Part model, mm, in its own coordinate system. A direction names the side the tool comes from. Coordinates: 2 decimals unless noted, no trailing zeros. Write each loop counter-clockwise with the first axis right and the second up, starting at its lowest first coordinate (ties: lowest second). Pieces come first, ordered by that corner, then holes. Notation, with made-up numbers: (19, -35.5) -> (67, -35.5) arc R20 ccw to (67, -15.5) -> close; hole circle Ø1 at (30.5, -8). An arc over 180 degrees is marked (long way). One line per question, with ' | ' between items. Start each with the question number.
Item 1: 3-axis set-ups, long thin cutter, end or side, ignore diameter. For faces 1 (the flat face through (0, 4, 18)), 2 (the cylindrical face through (-1.67, 6.17, 5.3)), 3 (the flat face through (3, 1.588, -3)): which of +Z, -Z, +X, -X, +Y, -Y reach the whole face in a straight line?
Item 2: Saw through at D-D (x = -14.5). List the corners of the cut face in (y, z).
Item 3: Saw through at A-A (x = 0). List the corners of the cut face in (y, z).
Item 4: Saw through at C-C (z = 0). List the corners of the cut face in (x, y).
Item 5: Probe probe 1 along Z at (x, y) = (12.7, 2); probe 2 along Z at (x, y) = (0, 2.25). List the from-to ranges inside material, lowest first. Write a range as [from, to].
Item 6: Two-plate mould, pull along X, no slides. Class faces 4 (the flat face through (-18, 4, 0)), 5 (the cylindrical face through (-13.375, 3.913, -10.556)), 6 (the flat face through (0, 7.938, 8)): pulls with the +X half, pulls with the -X half, needs draft (parallel to the pull), parting line crosses it, or undercut.
Item 7: Pin check, flat tips, straight feed: pin 1 (10 mm diameter, centred on x = 0, z = 0, fed in from +Y); pin 2 (2.5 mm diameter, centred on x = 12.7, z = 12.7, fed in from +Y). Stop position of each tip, or through.
Item 8: Saw through at B-B (y = 5.5). List the corners of the cut face in (x, z).
Autodesk Inventor part; units mm, degrees
ref_plane "YZ Plane" through (0, 0, 0) normal (1, 0, 0) x (0, 1, 0)
ref_plane "XZ Plane" through (0, 0, 0) normal (0, 1, 0) x (-1, 0, 0)
ref_plane "XY Plane" through (0, 0, 0) normal (0, 0, 1) x (1, 0, 0)
sketch "Sketch1" plane through (0, 0, 0) normal (0, 1, 0) x (-1, 0, 0)
  line L0 (-18, 18) -> (18, 18)
  line L1 (18, 18) -> (18, -18)
  line L2 (18, -18) -> (-18, -18)
  line L3 (-18, -18) -> (-18, 18)
  line L4 (-18, 18) -> (18, -18) construction
  line L5 (18, 18) -> (-18, -18) construction
  point P0 (0, 0)
  dimension "d0" = 36
  dimension "d1" = 36
extrude "Extrusion1" add sketch "Sketch1" along normal blind 7.9375
sketch "Sketch3" plane through (0, 7.9375, 0) normal (0, 1, 0) x (1, 0, 0)
  line L0 (-12.7, -12.7) -> (12.7, -12.7) construction
  line L1 (12.7, -12.7) -> (12.7, 12.7) construction
  line L2 (12.7, 12.7) -> (-12.7, 12.7) construction
  line L3 (-12.7, 12.7) -> (-12.7, -12.7) construction
  line L4 (-12.7, -12.7) -> (12.7, 12.7) construction
  line L5 (12.7, -12.7) -> (-12.7, 12.7) construction
  point P0 (0, 0)
  dimension "d11" = 25.4
hole "Hole2" at (-12.7, 7.9375, -12.7) at (12.7, 7.9375, -12.7) at (-12.7, 7.9375, 12.7) at (12.7, 7.9375, 12.7) direction (0, -1, 0) diameter 4.496 depth 12.3 tip angle 118
sketch "Sketch2" plane through (0, 7.9375, 0) normal (0, 1, 0) x (1, 0, 0)
  point P0 (0, 0)
  point P1 (0, 0)
hole "Hole1" at (0, 7.9375, 0) direction (0, -1, 0) diameter 6.528 end through all counterbore diameter 11.113 counterbore depth 3.25
fillet "Fillet1" radius 0.25 12 edges at (-18, 3.9688, 18) (0, 0, 18) (18, 3.9688, 18) (0, 7.9375, 18) (18, 7.9375, 0) (0, 7.9375, -18) (-18, 7.9375, 0) (18, 0, 0) (18, 3.9688, -18) (-18, 0, 0) (0, 0, -18) (-18, 3.9688, -18)
fillet "Fillet2" radius 0.25 1 edges at (0, 7.9375, -5.5565)
sketch "Sketch4" plane through (0, 0, 0) normal (0, -1, 0) x (1, 0, 0)
  circle A0 centre (0, 0) radius 12.687
  dimension "d21" = 25.374
extrude "Extrusion2" cut sketch "Sketch4" against normal blind 1.5875
properties part number "ball-holder-to-post-adapter" material "ABS Plastic"
From the geometry:
1) face 1: +Z, +X, -X, +Y, -Y | face 2: +Y | face 3: -Y
2) outline: (0, -17.75) arc R0.25 ccw to (0.25, -18) -> (7.69, -18) arc R0.25 ccw to (7.94, -17.75) -> (7.94, -14.05) -> (0, -14.05) -> close; (0, -11.35) -> (7.94, -11.35) -> (7.94, 11.35) -> (0, 11.35) -> close; (0, 14.05) -> (7.94, 14.05) -> (7.94, 17.75) arc R0.25 ccw to (7.69, 18) -> (0.25, 18) arc R0.25 ccw to (0, 17.75) -> close
3) outline: (0, -17.75) arc R0.25 ccw to (0.25, -18) -> (7.69, -18) arc R0.25 ccw to (7.94, -17.75) -> (7.94, -5.81) arc R0.25 ccw to (7.69, -5.56) -> (4.69, -5.56) -> (4.69, -3.26) -> (1.59, -3.26) -> (1.59, -12.69) -> (0, -12.69) -> close; (0, 12.69) -> (1.59, 12.69) -> (1.59, 3.26) -> (4.69, 3.26) -> (4.69, 5.56) -> (7.69, 5.56) arc R0.25 ccw to (7.94, 5.81) -> (7.94, 17.75) arc R0.25 ccw to (7.69, 18) -> (0.25, 18) arc R0.25 ccw to (0, 17.75) -> close
4) outline: (-18, 0.25) arc R0.25 ccw to (-17.75, 0) -> (-12.69, 0) -> (-12.69, 1.59) -> (-3.26, 1.59) -> (-3.26, 4.69) -> (-5.56, 4.69) -> (-5.56, 7.69) arc R0.25 ccw to (-5.81, 7.94) -> (-17.75, 7.94) arc R0.25 ccw to (-18, 7.69) -> close; (3.26, 1.59) -> (12.69, 1.59) -> (12.69, 0) -> (17.75, 0) arc R0.25 ccw to (18, 0.25) -> (18, 7.69) arc R0.25 ccw to (17.75, 7.94) -> (5.81, 7.94) arc R0.25 ccw to (5.56, 7.69) -> (5.56, 4.69) -> (3.26, 4.69) -> close
5) probe 1: [-18, -14.95], [-10.45, 10.45], [14.95, 18] | probe 2: [-18, -3.26], [3.26, 18]
6) face 4: pulls with the -X half | face 5: undercut | face 6: needs draft
7) pin 1: y = 4.69 | pin 2: through
8) outline: (-18, -17.75) arc R0.25 ccw to (-17.75, -18) -> (17.75, -18) arc R0.25 ccw to (18, -17.75) -> (18, 17.75) arc R0.25 ccw to (17.75, 18) -> (-17.75, 18) arc R0.25 ccw to (-18, 17.75) -> close; hole circle Ø4.5 at (-12.7, -12.7); hole circle Ø4.5 at (-12.7, 12.7); hole circle Ø11.11 at (0, 0); hole circle Ø4.5 at (12.7, -12.7); hole circle Ø4.5 at (12.7, 12.7)
